Design review of the part built by this model. Coordinates are the model's own, in mm. Face numbers are marked on the shaded views. A direction names the side the tool comes from. Coordinates: 2 decimals unless noted, no trailing zeros. Loops run counter-clockwise (first coordinate to the right, second up) from the corner with the lowest first, then second, coordinate; pieces in that order, holes last. Notation, with made-up numbers: M 17.25,45 L 70.25,45 A19 ccw 70.25,59 Z; hole C 73.5,21 d10. An arc over 180 degrees is marked long. One line per item, written item: value.
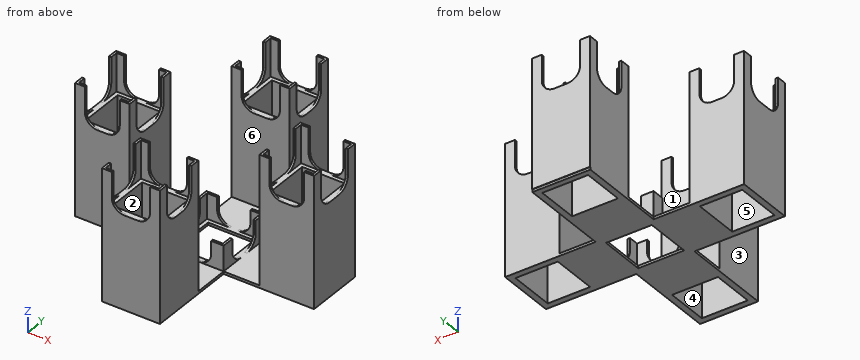
```python
from build123d import *

# Parameters (mm, degrees)
PAD_DEPTH     = 2
SKETCH001_W   = 43.2
SKETCH001_H   = 46
SKETCH001_W_2 = 46
SKETCH001_H_2 = 43.2
PAD001_DEPTH  = 71.7
PAD002_DEPTH  = 20
PAD003_DEPTH  = 30
SKETCH004_W   = 36.4
SKETCH004_H   = 33.6
SKETCH004_W_2 = 33.6
SKETCH004_H_2 = 36.4
POCKET_DEPTH  = 103.701
FILLET_R      = 10


with BuildPart() as part:
    # Sketch → Pad (new body)
    with BuildSketch(Plane.XY):
        Polygon((-51.5, 23), (-94.7, 23), (-94.7, -23), (-51.5, -23), (-23, -23), (-23, -51.5), (-23, -94.7), (23, -94.7), (23, -51.5), (23, -23), (51.5, -23), (94.7, -23), (94.7, 23), (51.5, 23), (23, 23), (23, 51.5), (23, 94.298633), (-23, 94.298633), (-23, 51.098633), (-23, 23), align=None)
    extrude(amount=PAD_DEPTH)

    # Sketch001 → Pad001 (new body)
    with BuildSketch(Plane.XY.offset(2)):
        with Locations((-73.1, 0)):
            Rectangle(SKETCH001_W, SKETCH001_H)
        with Locations((73.1, 0)):
            Rectangle(SKETCH001_W, SKETCH001_H)
        with Locations((0, 73.1)):
            Rectangle(SKETCH001_W_2, SKETCH001_H_2)
        with Locations((0, -73.1)):
            Rectangle(SKETCH001_W_2, SKETCH001_H_2)
    extrude(amount=PAD001_DEPTH)

    # Sketch002 → Pad002 (new body)
    with BuildSketch(Plane.XY.offset(2)):
        Polygon((-23, 23), (-23, 13.2), (-21.2, 13.2), (-21.2, 21.2), (-13.2, 21.2), (-13.2, 23), align=None)
        Polygon((21.2, 21.2), (13.2, 21.2), (13.2, 23), (23, 23), (23, 13.2), (21.2, 13.2), align=None)
        Polygon((23, -23), (23, -13.2), (21.2, -13.2), (21.2, -21.2), (13.2, -21.2), (13.2, -23), align=None)
        Polygon((-21.2, -21.2), (-21.2, -13.2), (-23, -13.2), (-23, -23), (-13.2, -23), (-13.2, -21.2), align=None)
    extrude(amount=PAD002_DEPTH)

    # Sketch003 → Pad003 (new body)
    with BuildSketch(Plane.XY.offset(73.7)):
        Polygon((-94.7, 23), (-94.7, 15.2), (-92.9, 15.2), (-92.9, 21.2), (-86.9, 21.2), (-86.9, 23), align=None)
        Polygon((-51.5, 23), (-59.3, 23), (-59.3, 21.2), (-53.3, 21.2), (-53.3, 15.2), (-51.5, 15.2), align=None)
        Polygon((-92.9, -15.2), (-92.9, -21.2), (-86.9, -21.2), (-86.9, -23), (-94.7, -23), (-94.7, -15.2), align=None)
        Polygon((-51.5, -23), (-51.5, -15.2), (-53.3, -15.2), (-53.3, -21.2), (-59.3, -21.2), (-59.3, -23), align=None)
        Polygon((-23, -59.3), (-23, -51.5), (-15.2, -51.5), (-15.2, -53.3), (-21.2, -53.3), (-21.2, -59.3), align=None)
        Polygon((-23, -94.7), (-23, -86.9), (-21.2, -86.9), (-21.2, -92.9), (-15.2, -92.9), (-15.2, -94.7), align=None)
        Polygon((15.2, -51.5), (23, -51.5), (23, -59.3), (21.2, -59.3), (21.2, -53.3), (15.2, -53.3), align=None)
        Polygon((23, -94.7), (15.2, -94.7), (15.2, -92.9), (21.2, -92.9), (21.2, -86.9), (23, -86.9), align=None)
        Polygon((51.5, 23), (51.5, 15.2), (53.3, 15.2), (53.3, 21.2), (59.3, 21.2), (59.3, 23), align=None)
        Polygon((94.7, 23), (86.9, 23), (86.9, 21.2), (92.9, 21.2), (92.9, 15.2), (94.7, 15.2), align=None)
        Polygon((51.5, -23), (51.5, -15.2), (53.3, -15.2), (53.3, -21.2), (59.3, -21.2), (59.3, -23), align=None)
        Polygon((94.7, -23), (86.9, -23), (86.9, -21.2), (92.9, -21.2), (92.9, -15.2), (94.7, -15.2), align=None)
        Polygon((-23, 51.5), (-23, 59.3), (-21.2, 59.3), (-21.2, 53.3), (-15.2, 53.3), (-15.2, 51.5), align=None)
        Polygon((15.2, 51.5), (15.2, 53.3), (21.2, 53.3), (21.2, 59.3), (23, 59.3), (23, 51.5), align=None)
        Polygon((15.2, 94.7), (23, 94.7), (23, 86.9), (21.2, 86.9), (21.2, 92.9), (15.2, 92.9), align=None)
        Polygon((-15.2, 94.7), (-15.2, 92.9), (-21.2, 92.9), (-21.2, 86.9), (-23, 86.9), (-23, 94.7), align=None)
    extrude(amount=PAD003_DEPTH)

    # Sketch004 → Pocket (cut, through all)
    with BuildSketch(Plane(origin=(0, 0, 0), x_dir=(1, 0, 0), z_dir=(0, 0, -1))):
        with Locations((0, 73.1)):
            Rectangle(SKETCH004_W, SKETCH004_H)
        with Locations((0, -73.1)):
            Rectangle(SKETCH004_W, SKETCH004_H)
        with Locations((-73.1, 0)):
            Rectangle(SKETCH004_W_2, SKETCH004_H_2)
        with Locations((73.1, 0)):
            Rectangle(SKETCH004_W_2, SKETCH004_H_2)
        Rectangle(SKETCH004_W, SKETCH004_H_2)
    extrude(amount=-POCKET_DEPTH, mode=Mode.SUBTRACT)

    # Fillet
    fillet_edges = [part.edges().sort_by_distance(p)[0] for p in [
        (15.2, 93.8, 73.7),
        (15.2, 52.4, 73.7),
        (15.2, -52.4, 73.7),
        (15.2, -93.8, 73.7),
        (86.9, -22.1, 73.7),
        (86.9, 22.1, 73.7),
        (-59.3, -22.1, 73.7),
        (-59.3, 22.1, 73.7),
        (22.1, 59.3, 73.7),
        (-22.1, 59.3, 73.7),
        (-93.8, -15.2, 73.7),
        (-52.4, -15.2, 73.7),
        (-22.1, -86.9, 73.7),
        (22.1, -86.9, 73.7),
        (52.4, -15.2, 73.7),
        (93.8, -15.2, 73.7),
        (-15.2, -93.8, 73.7),
        (-15.2, -52.4, 73.7),
        (-86.9, -22.1, 73.7),
        (-86.9, 22.1, 73.7),
        (-15.2, 52.4, 73.7),
        (-15.2, 93.8, 73.7),
        (59.3, 22.1, 73.7),
        (59.3, -22.1, 73.7),
        (-22.1, 86.9, 73.7),
        (22.1, 86.9, 73.7),
        (52.4, 15.2, 73.7),
        (93.8, 15.2, 73.7),
        (22.1, -59.3, 73.7),
        (-22.1, -59.3, 73.7),
        (-52.4, 15.2, 73.7),
        (-93.8, 15.2, 73.7),
        (13.2, -22.1, 2),
        (22.1, -13.2, 2),
        (22.1, 13.2, 2),
        (-22.1, 13.2, 2),
        (13.2, 22.1, 2),
        (-13.2, 22.1, 2),
        (-13.2, -22.1, 2),
        (-22.1, -13.2, 2),
    ]]
    fillet(fillet_edges, radius=FILLET_R)


solid = part.part
```
(1) We need section B-B on z = 37. State how many separate pieces and enclosed holes the cut face has, then the cut area to 3 significant figures.
Reply:
separate pieces: 4
enclosed holes: 4
area: 3,060 mm2
(2) Mouldability with a two-part tool opening along X and no side actions: class the marked faces 3, 4, 5 and 6 as released by +X, released by -X, zero draft, split by the parting line, or undercut.
Reply:
face 3: released by -X
face 4: undercut
face 5: undercut
face 6: zero draft
(3) Insertion check: pin 1 (5 mm diameter, centred on x = 61.5, z = 92, fed in from -Y); pin 2 (12 mm diameter, centred on y = -71.5, z = 24.5, fed in from +X); pin 3 (5 mm diameter, centred on x = -59, z = 92, fed in from +Y); pin 4 (8 mm diameter, centred on x = 13.5, z = 87, fed in from +Y). Each pin has a flat end and moves straight along its axis. Give the tip position at first contact, or say it passes through.
Reply:
pin 1: stops at y = -23
pin 2: stops at x = 23
pin 3: stops at y = 23
pin 4: stops at y = 94.7
(4) To check wall thickness, follow line 1 along X through (y, z) = (-14, 50.5); line 2 along X through (y, z) = (-20, 91.5). State the ranges of each line that lie inside material, in increasing order. Write a range as [from, to].
Reply:
line 1: x = [-94.7, -89.9], [-56.3, -51.5], [51.5, 56.3], [89.9, 94.7]
line 2: x = [-94.7, -92.9], [-53.3, -51.5], [51.5, 53.3], [92.9, 94.7]
(5) We need section A-A on y = -72. State the section outline as (x, z) points.
Reply:
outline: M -23,0 L -18.2,0 L -18.2,73.7 L -23,73.7 Z; M 18.2,0 L 23,0 L 23,73.7 L 18.2,73.7 Z
(6) We need section D-D on x = -82.5. State the section outline as (y, z) points, then the cut area to 3 significant figures.
Reply:
outline: M -23,0 L -18.2,0 L -18.2,73.7 L -21.2,73.7 L -21.2,75.42 L -23,75.42 Z; M 18.2,0 L 23,0 L 23,75.42 L 21.2,75.42 L 21.2,73.7 L 18.2,73.7 Z
area: 714 mm2
(7) Tool access review of the marked faces 1 and 2: name each direction out of +Z, -Z, +X, -X, +Y, -Y from which nothing blocks a thin tool from reaching the whole face with its end or side.
Reply:
face 1: +Z, +X, -X
face 2: +Z, -Z
